```python
from build123d import *

# Parameters (mm, degrees)
SKETCH_2_R          = 4
SKETCH_2_R_2        = 3.4
EXTRUDE_1_DEPTH     = 580
SKETCH_3_R          = 5.341354258
SKETCH_3_R_2        = 5.383492222
SKETCH_3_R_3        = 4.933832051
SKETCH_3_R_4        = 5.418030405
SKETCH_3_R_5        = 5.574298651
EXTRUDE_2_DEPTH     = 580
SKETCH_4_R          = 4
CUT_EXTRUDE_1_DEPTH = 581


with BuildPart() as part:
    # 草图2 → 凸台-拉伸1 (new body)
    with BuildSketch(Plane(origin=(0, 0, 0), x_dir=(1, 0, 0), z_dir=(0, 1, 0))):
        with BuildLine():
            Line((212.330022346, 152.083698324), (201.421584322, 152.083698324))
            ThreePointArc((201.421584322, 152.083698324), (186.766061316, 142.219737293), (196.630022346, 156.8752603))
            Line((196.630022346, 156.8752603), (196.630022346, 167.783698324))
            Line((196.630022346, 167.783698324), (193.130022346, 167.783698324))
            Line((193.130022346, 167.783698324), (193.130022346, 164.833698324))
            Line((193.130022346, 164.833698324), (185.630022346, 164.833698324))
            ThreePointArc((185.630022346, 164.833698324), (182.630022346, 172.083698324), (185.630022346, 179.333698324))
            Line((185.630022346, 179.333698324), (193.130022346, 179.333698324))
            Line((193.130022346, 179.333698324), (193.130022346, 176.383698324))
            Line((193.130022346, 176.383698324), (196.630022346, 176.383698324))
            Line((196.630022346, 176.383698324), (196.630022346, 191.583698324))
            ThreePointArc((196.630022346, 191.583698324), (196.483575737, 191.937251715), (196.130022346, 192.083698324))
            Line((196.130022346, 192.083698324), (180.930022346, 192.083698324))
            Line((180.930022346, 192.083698324), (180.930022346, 188.583698324))
            Line((180.930022346, 188.583698324), (183.880022346, 188.583698324))
            Line((183.880022346, 188.583698324), (183.880022346, 181.083698324))
            ThreePointArc((183.880022346, 181.083698324), (176.630022346, 178.083698324), (169.380022346, 181.083698324))
            Line((169.380022346, 181.083698324), (169.380022346, 188.583698324))
            Line((169.380022346, 188.583698324), (172.330022346, 188.583698324))
            Line((172.330022346, 188.583698324), (172.330022346, 192.083698324))
            Line((172.330022346, 192.083698324), (157.130022346, 192.083698324))
            ThreePointArc((157.130022346, 192.083698324), (156.776468956, 191.937251715), (156.630022346, 191.583698324))
            Line((156.630022346, 191.583698324), (156.630022346, 176.383698324))
            Line((156.630022346, 176.383698324), (160.130022346, 176.383698324))
            Line((160.130022346, 176.383698324), (160.130022346, 179.333698324))
            Line((160.130022346, 179.333698324), (167.630022346, 179.333698324))
            ThreePointArc((167.630022346, 179.333698324), (170.630022346, 172.083698324), (167.630022346, 164.833698324))
            Line((167.630022346, 164.833698324), (160.130022346, 164.833698324))
            Line((160.130022346, 164.833698324), (160.130022346, 167.783698324))
            Line((160.130022346, 167.783698324), (156.630022346, 167.783698324))
            Line((156.630022346, 167.783698324), (156.630022346, 136.383698324))
            Line((156.630022346, 136.383698324), (160.130022346, 136.383698324))
            Line((160.130022346, 136.383698324), (160.130022346, 139.333698324))
            Line((160.130022346, 139.333698324), (167.630022346, 139.333698324))
            ThreePointArc((167.630022346, 139.333698324), (170.630022346, 132.083698324), (167.630022346, 124.833698324))
            Line((167.630022346, 124.833698324), (160.130022346, 124.833698324))
            Line((160.130022346, 124.833698324), (160.130022346, 127.783698324))
            Line((160.130022346, 127.783698324), (156.630022346, 127.783698324))
            Line((156.630022346, 127.783698324), (156.630022346, 112.583698324))
            ThreePointArc((156.630022346, 112.583698324), (156.776468956, 112.230144933), (157.130022346, 112.083698324))
            Line((157.130022346, 112.083698324), (172.330022346, 112.083698324))
            Line((172.330022346, 112.083698324), (172.330022346, 115.583698324))
            Line((172.330022346, 115.583698324), (169.380022346, 115.583698324))
            Line((169.380022346, 115.583698324), (169.380022346, 123.083698324))
            ThreePointArc((169.380022346, 123.083698324), (176.630022346, 126.083698324), (183.880022346, 123.083698324))
            Line((183.880022346, 123.083698324), (183.880022346, 115.583698324))
            Line((183.880022346, 115.583698324), (180.930022346, 115.583698324))
            Line((180.930022346, 115.583698324), (180.930022346, 112.083698324))
            Line((180.930022346, 112.083698324), (196.130022346, 112.083698324))
            Line((196.130022346, 112.083698324), (212.330022346, 112.083698324))
            Line((212.330022346, 112.083698324), (212.330022346, 115.583698324))
            Line((212.330022346, 115.583698324), (209.380022346, 115.583698324))
            Line((209.380022346, 115.583698324), (209.380022346, 123.083698324))
            ThreePointArc((209.380022346, 123.083698324), (216.630022346, 126.083698324), (223.880022346, 123.083698324))
            Line((223.880022346, 123.083698324), (223.880022346, 115.583698324))
            Line((223.880022346, 115.583698324), (220.930022346, 115.583698324))
            Line((220.930022346, 115.583698324), (220.930022346, 112.083698324))
            Line((220.930022346, 112.083698324), (236.130022346, 112.083698324))
            ThreePointArc((236.130022346, 112.083698324), (236.483575737, 112.230144933), (236.630022346, 112.583698324))
            Line((236.630022346, 112.583698324), (236.630022346, 127.783698324))
            Line((236.630022346, 127.783698324), (233.130022346, 127.783698324))
            Line((233.130022346, 127.783698324), (233.130022346, 124.833698324))
            Line((233.130022346, 124.833698324), (225.630022346, 124.833698324))
            ThreePointArc((225.630022346, 124.833698324), (222.630022346, 132.083698324), (225.630022346, 139.333698324))
            Line((225.630022346, 139.333698324), (233.130022346, 139.333698324))
            Line((233.130022346, 139.333698324), (233.130022346, 136.383698324))
            Line((233.130022346, 136.383698324), (236.630022346, 136.383698324))
            Line((236.630022346, 136.383698324), (236.630022346, 151.583698324))
            ThreePointArc((236.630022346, 151.583698324), (236.483575737, 151.937251715), (236.130022346, 152.083698324))
            Line((236.130022346, 152.083698324), (220.930022346, 152.083698324))
            Line((220.930022346, 152.083698324), (220.930022346, 148.583698324))
            Line((220.930022346, 148.583698324), (223.880022346, 148.583698324))
            Line((223.880022346, 148.583698324), (223.880022346, 141.083698324))
            ThreePointArc((223.880022346, 141.083698324), (216.630022346, 138.083698324), (209.380022346, 141.083698324))
            Line((209.380022346, 141.083698324), (209.380022346, 148.583698324))
            Line((209.380022346, 148.583698324), (212.330022346, 148.583698324))
            Line((212.330022346, 148.583698324), (212.330022346, 152.083698324))
        make_face()
        with Locations((162.630022346, 118.083698324)):
            Circle(SKETCH_2_R, mode=Mode.SUBTRACT)
        with BuildLine():
            ThreePointArc((206.380022346, 118.583698324), (205.50134269, 116.46237798), (203.380022346, 115.583698324))
            Line((203.380022346, 115.583698324), (186.880022346, 115.583698324))
            Line((186.880022346, 115.583698324), (186.880022346, 124.236137901))
            ThreePointArc((186.880022346, 124.236137901), (184.480651994, 126.510014755), (181.593404213, 128.119764513))
            ThreePointArc((181.593404213, 128.119764513), (180.080209042, 129.469558022), (179.77133004, 131.473627856))
            ThreePointArc((179.77133004, 131.473627856), (174.367280647, 129.820956624), (176.019951879, 135.225006017))
            ThreePointArc((176.019951879, 135.225006017), (174.015882044, 135.53388502), (172.666088535, 137.047080191))
            ThreePointArc((172.666088535, 137.047080191), (171.056338777, 139.934327972), (168.782461923, 142.333698324))
            Line((168.782461923, 142.333698324), (163.130022346, 142.333698324))
            ThreePointArc((163.130022346, 142.333698324), (161.008702003, 143.21237798), (160.130022346, 145.333698324))
            Line((160.130022346, 145.333698324), (160.130022346, 158.833698324))
            ThreePointArc((160.130022346, 158.833698324), (161.008702003, 160.955018668), (163.130022346, 161.833698324))
            Line((163.130022346, 161.833698324), (169.130022346, 161.833698324))
            Line((169.130022346, 161.833698324), (175.130022346, 166.583698324))
            Line((175.130022346, 166.583698324), (178.130022346, 166.583698324))
            Line((178.130022346, 166.583698324), (184.130022346, 161.833698324))
            Line((184.130022346, 161.833698324), (190.130022346, 161.833698324))
            ThreePointArc((190.130022346, 161.833698324), (191.967307675, 161.205276411), (193.034866096, 159.583286739))
            ThreePointArc((193.034866096, 159.583286739), (185.351847753, 140.805523731), (204.129610761, 148.488542073))
            ThreePointArc((204.129610761, 148.488542073), (205.751600433, 147.420983653), (206.380022346, 145.583698324))
            Line((206.380022346, 145.583698324), (206.380022346, 139.583698324))
            Line((206.380022346, 139.583698324), (211.130022346, 133.583698324))
            Line((211.130022346, 133.583698324), (211.130022346, 130.583698324))
            Line((211.130022346, 130.583698324), (206.380022346, 124.583698324))
            Line((206.380022346, 124.583698324), (206.380022346, 118.583698324))
        make_face(mode=Mode.SUBTRACT)
        with Locations((230.630022346, 118.083698324)):
            Circle(SKETCH_2_R, mode=Mode.SUBTRACT)
        with Locations((216.630022346, 132.083698324)):
            Circle(SKETCH_2_R_2, mode=Mode.SUBTRACT)
        with Locations((230.130022346, 145.583698324)):
            Circle(SKETCH_2_R, mode=Mode.SUBTRACT)
        with Locations((176.630022346, 172.083698324)):
            Circle(SKETCH_2_R_2, mode=Mode.SUBTRACT)
        with Locations((163.130022346, 186.083698324)):
            Circle(SKETCH_2_R, mode=Mode.SUBTRACT)
        with Locations((190.130022346, 185.583698324)):
            Circle(SKETCH_2_R, mode=Mode.SUBTRACT)
    extrude(amount=EXTRUDE_1_DEPTH)

    # 草图3 → 凸台-拉伸2 (add)
    with BuildSketch(Plane(origin=(0, 580, 0), x_dir=(1, 0, 0), z_dir=(0, 1, 0))):
        with Locations((163.130022346, 186.083698324)):
            Circle(SKETCH_3_R)
        with Locations((190.130022346, 185.583698324)):
            Circle(SKETCH_3_R_2)
        with Locations((162.630022346, 118.083698324)):
            Circle(SKETCH_3_R_3)
        with Locations((230.630022346, 118.083698324)):
            Circle(SKETCH_3_R_4)
        with Locations((230.130022346, 145.583698324)):
            Circle(SKETCH_3_R_5)
    extrude(amount=-EXTRUDE_2_DEPTH)

    # 草图4 → 切除-拉伸1 (cut, through all)
    with BuildSketch(Plane(origin=(0, 580, 0), x_dir=(1, 0, 0), z_dir=(0, 1, 0))):
        with Locations((163.130022346, 185.583698324)):
            Circle(SKETCH_4_R)
        with Locations((163.130022346, 118.583698324)):
            Circle(SKETCH_4_R)
        with Locations((230.130022346, 118.583698324)):
            Circle(SKETCH_4_R)
        with Locations((230.130022346, 145.583698324)):
            Circle(SKETCH_4_R)
        with Locations((190.130022346, 185.583698324)):
            Circle(SKETCH_4_R)
    extrude(amount=-CUT_EXTRUDE_1_DEPTH, mode=Mode.SUBTRACT)


solid = part.part
```
Input: part model. Units: mm. Frame: model coordinates. A direction names the side the tool comes from. Round coordinates to 2 decimals unless told otherwise and drop trailing zeros. One line per item, written item: value. Start each with the question number.
(1) Ray query, line 1 (Z direction, x = 230, y = 181.5); line 2 (X direction, y = 284, z = -185); line 3 (Z direction, x = 217, y = 377). Return the intervals inside material, ascending. Write a range as [from, to].
(2) Section A-A, the plane y = 423. Count the separate pieces of the cut face and the enclosed holes in it, plus the area to 3 significant figures.
(3) Contact query for flat-ended pins moving along their axis: P1, Ø8.5, axis at x = 209, y = 164, coming from the -Z side; P2, Ø1.5, axis at y = 186, z = -172.5, coming from the +X side; P3, Ø3.5, axis at x = 177.5, y = 206.5, coming from the +Z side. Output: stop coordinate, or through.
(4) Access query for faces 4 (the flat face through (207, 286, -152.084)), 5 (the flat face through (195, 286, -115.584)), 6 (the flat face through (236.63, 286, -120)). Directions: +Z, -Z, +X, -X, +Y, -Y. A direction counts if a zero-diameter tool reaches every point of the face in a straight line with its end or side. Return the directions, or none.
(5) Draft query along X for faces 1 (the flat face through (196.63, 286, -184)), 2 (the flat face through (165, 286, -192.084)), 3 (the flat face through (160.13, 286, -152)). Return one class per face: +X half, -X half, draft (parallel to the pull), parting line (faces both ways), or undercut.
Results below:
1. line 1: [-152.08, -149.58], [-141.59, -139.33], [-124.83, -122.58], [-114.59, -112.08]
1. line 2: [156.63, 159.17], [167.09, 169.38], [183.88, 186.17], [194.09, 196.63]
1. line 3: [-138.09, -135.46], [-128.7, -126.08]
2. separate pieces: 1
2. enclosed holes: 8
2. area: 1,650 mm^2
3. P1: z = -152.08
3. P2: x = 182.7
3. P3: z = -125.74
4. face 4: -Z, +X, +Y, -Y
4. face 5: +Y, -Y
4. face 6: +Z, -Z, +X, +Y, -Y
5. face 1: +X half
5. face 2: draft
5. face 3: undercut
